from build123d import *

# Parameters (mm, degrees)
SKETCH_1_R                  = 19
EXTRUDE_1_DEPTH             = 3
SKETCH_2_R                  = 1.05
CUT_EXTRUDE_1_DEPTH         = 28.037011669
SKETCH_3_R                  = 7
EXTRUDE_2_DEPTH             = 9.8
SKETCH_4_R                  = 17
EXTRUDE_3_DEPTH             = 3
HOLE_WIZARD_3_2_3_2_1_D     = 3.2
HOLE_WIZARD_3_2_3_2_1_DEPTH = 6
HOLE_WIZARD_3_2_3_2_1_TIP   = 0.96137699
SKETCH_7_R                  = 3
CUT_EXTRUDE_2_DEPTH         = 4
SKETCH_8_R                  = 2.05
CUT_EXTRUDE_3_DEPTH         = 4


with BuildPart() as part:
    # 草图1 → 凸台-拉伸1 (new body)
    with BuildSketch(Plane.XY):
        Circle(SKETCH_1_R)
    extrude(amount=EXTRUDE_1_DEPTH)

    # 草图2 → 切除-拉伸1 (cut, through all)
    with BuildSketch(Plane.XY.offset(3)):
        with Locations((0, 12.5)):
            Circle(SKETCH_2_R)
        with Locations((-9.5, 0)):
            Circle(SKETCH_2_R)
        with Locations((9.5, 0)):
            Circle(SKETCH_2_R)
        with Locations((0, -12.5)):
            Circle(SKETCH_2_R)
        with Locations((-2.77644219, 15.757264)):
            Circle(SKETCH_2_R)
        with Locations((15.034412013, -5.474162531)):
            Circle(SKETCH_2_R)
        with Locations((-12.257969823, -10.283101469)):
            Circle(SKETCH_2_R)
    extrude(amount=-CUT_EXTRUDE_1_DEPTH, mode=Mode.SUBTRACT)

    # 草图3 → 凸台-拉伸2 (add)
    with BuildSketch(Plane.XY.offset(3)):
        Circle(SKETCH_3_R)
    extrude(amount=EXTRUDE_2_DEPTH)

    # 草图4 → 凸台-拉伸3 (add)
    with BuildSketch(Plane.XY.offset(12.8)):
        Circle(SKETCH_4_R)
    extrude(amount=EXTRUDE_3_DEPTH)

    # Ø3.2 (3.2) 直径孔1
    with Locations(Plane.XY.offset(15.8)):
        with Locations((0, 0)):
            Hole(HOLE_WIZARD_3_2_3_2_1_D / 2, depth=HOLE_WIZARD_3_2_3_2_1_DEPTH)
            with Locations((0, 0, -(HOLE_WIZARD_3_2_3_2_1_DEPTH + HOLE_WIZARD_3_2_3_2_1_TIP / 2))):  # 118° drill point
                Cone(0, HOLE_WIZARD_3_2_3_2_1_D / 2, HOLE_WIZARD_3_2_3_2_1_TIP, mode=Mode.SUBTRACT)

    # 草图7 → 切除-拉伸2 (cut)
    with BuildSketch(Plane(origin=(0, 0, 0), x_dir=(-1, 0, 0), z_dir=(0, 0, -1))):
        Circle(SKETCH_7_R)
    extrude(amount=-CUT_EXTRUDE_2_DEPTH, mode=Mode.SUBTRACT)

    # 草图8 → 切除-拉伸3 (cut)
    with BuildSketch(Plane.XY.offset(15.8)):
        with Locations((8.838834765, 8.838834765)):
            Circle(SKETCH_8_R)
        with Locations((8.838834765, -8.838834765)):
            Circle(SKETCH_8_R)
        with Locations((-8.838834765, -8.838834765)):
            Circle(SKETCH_8_R)
        with Locations((-8.838834765, 8.838834765)):
            Circle(SKETCH_8_R)
    extrude(amount=-CUT_EXTRUDE_3_DEPTH, mode=Mode.SUBTRACT)


solid = part.part
Can you work these out from the model? Positions are in its coordinate system, mm. A direction names the side the tool comes from. Give positions to 0.01 mm unless a question says otherwise; leave off trailing zeros. Loops run counter-clockwise (first coordinate to the right, second up) from the corner with the lowest first, then second, coordinate; pieces in that order, holes last. Notation, with made-up numbers: (75.5, 24) -> (128.5, 24) arc R34 ccw to (128.5, 62) -> close; hole circle Ø1 at (21, 76). An arc over 180 degrees is marked (long way). Use one line per item in the form item = value.
1) If we section it at B-B (y = -16): Please give me the cut outline in (x, z), plus the area to 3 significant figures.
Answers:
outline = (-10.25, 0) -> (10.25, 0) -> (10.25, 3) -> (-10.25, 3) -> close; (-5.74, 12.8) -> (5.74, 12.8) -> (5.74, 15.8) -> (-5.74, 15.8) -> close
area = 95.9 mm²
2) I need wall thicknesses on line 1 along Y through (x, z) = (0, 1.5); line 2 along Z through (x, y) = (-7, -2); line 3 along Y through (x, z) = (0, 13.5). Which ranges of each line are inside material? Lowest first, please.
Answers:
line_1 = -19 to -13.55, -11.45 to -3, 3 to 11.45, 13.55 to 19
line_2 = 0 to 3, 12.8 to 15.8
line_3 = -17 to -1.6, 1.6 to 17
3) For faces 1 (the face through (6.79, 8.93, 14.32)), 2 (the face through (8, 0, 3)), 3 (the face through (-8.5, 0.32, 1.52)), which set-ups out of +Z, -Z, +X, -X, +Y, -Y let a thin tool reach every point of the face, with its end or its side?
Answers:
face_1 = +Z
face_2 = none
face_3 = -Z
4) If we section it at A-A (x = 8): Please give me the cut outline in (y, z), plus the area to 3 significant figures.
Answers:
outline = (-17.23, 0) -> (17.23, 0) -> (17.23, 3) -> (-17.23, 3) -> close; (-15, 12.8) -> (-10.71, 12.8) -> (-10.71, 15.8) -> (-15, 15.8) -> close; (-6.97, 12.8) -> (6.97, 12.8) -> (6.97, 15.8) -> (-6.97, 15.8) -> close; (10.71, 12.8) -> (15, 12.8) -> (15, 15.8) -> (10.71, 15.8) -> close
area = 171 mm²
5) Will these pins go through, and if not, where does the flat tip stop? pin 1 (4 mm diameter, centred on y = 3.5, z = 3.5, fed in from +X); pin 2 (1.9 mm diameter, centred on x = -9.5, y = 0, fed in from -Z); pin 3 (2.5 mm diameter, centred on x = 0, y = 0, fed in from +Z).
Answers:
pin_1 = 18.94
pin_2 = 12.8
pin_3 = 9.59
6) If we section it at C-C (x = 15.5): Please give me the cut outline in (y, z), plus the area to 3 significant figures.
Answers:
outline = (-10.99, 0) -> (-6.42, 0) -> (-6.42, 3) -> (-10.99, 3) -> close; (-6.98, 12.8) -> (6.98, 12.8) -> (6.98, 15.8) -> (-6.98, 15.8) -> close; (-4.53, 0) -> (10.99, 0) -> (10.99, 3) -> (-4.53, 3) -> close
area = 102 mm²
7) We'd pull the mould along Y, two halves only. Please class faces 4 (the face through (6.79, -8.75, 14.32)), 5 (the face through (4, 0, 0)), 6 (the face through (6.466, -2.681, 7.831)): released by +Y, released by -Y, zero draft, split by the parting line, or undercut.
Answers:
face_4 = undercut
face_5 = zero draft
face_6 = split by the parting line
